CAD build for the part. Positions are in the model's coordinates, mm. Face numbers are marked on the shaded views. A direction names the side the tool comes from. Coordinates: 2 decimals unless noted, no trailing zeros. Loops run counter-clockwise (first coordinate to the right, second up) from the corner with the lowest first, then second, coordinate; pieces in that order, holes last. Notation, with made-up numbers: (-11.75, 58) -> (-0.75, 58) arc R21 cw to (-0.75, 92) -> close; hole circle Ø8 at (-33.75, -33). An arc over 180 degrees is marked (long way). Return JSON: item names as keys, results as strings. Group by question number.
(1) Tool access for the marked faces 1 and 2: list every direction of +Z, -Z, +X, -X, +Y, -Y with a clear straight run to the whole face (end or side of a thin tool).
(2) Saw through at C-C on y = 25.25. Write the cut outline in (x, z), then the cut area to 3 significant figures.
(3) Saw through at D-D on y = 12.25. Write the cut outline in (x, z), then the cut area to 3 significant figures.
(4) Saw through at A-A on x = 5. Write the cut outline in (y, z).
(5) Saw through at B-B on z = 1.5. Write the cut outline in (x, y).
(6) Flat gauge pin, fed straight in: pin 1 Ø1.5 at (x, y) = (1.5, 24.5) entering from +Z. Where does the tip first touch, or does it go through?
(7) Probe L1, parallel to Y at x = 5, z = 1.45; L2, parallel to Z at x = 8.5, y = 22.5; L3, parallel to Y at x = 5.25, z = 8.5. List the from-to ranges inside material, lowest first.
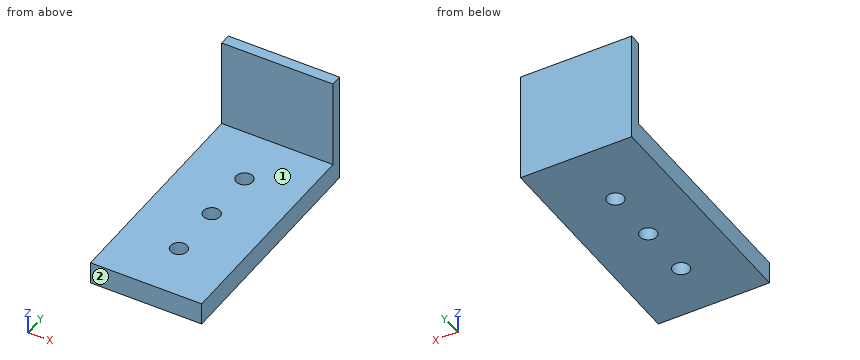
```python
from build123d import *

# Parameters (mm, degrees)
SKETCH1_W           = 10
SKETCH1_H           = 20
BOSS_EXTRUDE1_DEPTH = 2
SKETCH2_R           = 0.75
CUT_EXTRUDE2_DEPTH  = 2
SKETCH5_W           = 10
SKETCH5_H           = 10
BOSS_EXTRUDE2_DEPTH = 1


with BuildPart() as part:
    # Sketch1 → Boss-Extrude1 (new body)
    with BuildSketch(Plane.XY):
        with Locations((5, 19.715051701)):
            Rectangle(SKETCH1_W, SKETCH1_H)
    extrude(amount=BOSS_EXTRUDE1_DEPTH)

    # Sketch2 → Cut-Extrude2 (cut)
    with BuildSketch(Plane.XY):
        with Locations((5, 24.715051701)):
            Circle(SKETCH2_R)
        with Locations((5, 19.715051701)):
            Circle(SKETCH2_R)
        with Locations((5, 14.715051701)):
            Circle(SKETCH2_R)
    extrude(amount=CUT_EXTRUDE2_DEPTH, mode=Mode.SUBTRACT)

    # Sketch5 → Boss-Extrude2 (add)
    with BuildSketch(Plane(origin=(0, 29.715051701, 0), x_dir=(1, 0, 0), z_dir=(0, 1, 0))):
        with Locations((5, -5)):
            Rectangle(SKETCH5_W, SKETCH5_H)
    extrude(amount=BOSS_EXTRUDE2_DEPTH)


solid = part.part
```
Geometry results:
{
 "1": {"face 1": "+Z, +X, -X, -Y", "face 2": "+Z, -Z, +X, -X, -Y"},
 "2": {"outline": "(0, 0) -> (4.47, 0) -> (4.47, 2) -> (0, 2) -> close; (5.53, 0) -> (10, 0) -> (10, 2) -> (5.53, 2) -> close", "area": "17.9 mm²"},
 "3": {"outline": "(0, 0) -> (10, 0) -> (10, 2) -> (0, 2) -> close", "area": "20.0 mm²"},
 "4": {"outline": "(9.72, 0) -> (13.97, 0) -> (13.97, 2) -> (9.72, 2) -> close; (15.47, 0) -> (18.97, 0) -> (18.97, 2) -> (15.47, 2) -> close; (20.47, 0) -> (23.97, 0) -> (23.97, 2) -> (20.47, 2) -> close; (25.47, 0) -> (30.72, 0) -> (30.72, 10) -> (29.72, 10) -> (29.72, 2) -> (25.47, 2) -> close"},
 "5": {"outline": "(0, 9.72) -> (10, 9.72) -> (10, 30.72) -> (0, 30.72) -> close; hole circle Ø1.5 at (5, 14.72); hole circle Ø1.5 at (5, 19.72); hole circle Ø1.5 at (5, 24.72)"},
 "6": {"pin 1": "z = 2"},
 "7": {"L1": "9.72 to 13.97, 15.47 to 18.97, 20.47 to 23.97, 25.47 to 30.72", "L2": "0 to 2", "L3": "29.72 to 30.72"}
}
